from build123d import *

# Parameters (mm, degrees)
EXTRUDE_1_DEPTH     = 42.5
SKETCH_2_OUTSIDE_W  = 122.554
SKETCH_2_OUTSIDE_H  = 44.054
CUT_EXTRUDE_1_DEPTH = 78
SKETCH_3_W          = 40
SKETCH_3_H          = 40
CUT_EXTRUDE_2_DEPTH = 7.5
SKETCH_4_W          = 152
SKETCH_4_H          = 82
CUT_EXTRUDE_3_DEPTH = 2


with BuildPart() as part:
    # Эскиз1 → Бобышка-Вытянуть1 (new body, symmetric)
    with BuildSketch(Plane.XY):
        Polygon((0, 0), (-78, 0), (-78, 2.705180544), (-60.423159652, 6.5), (-10.423159652, 6.5), (0, 2.705180544), (10.423159652, 6.5), (60.423159652, 6.5), (78, 2.705180544), (78, 0), align=None)
    extrude(amount=EXTRUDE_1_DEPTH, both=True)

    # Эскиз2 outside → Вырез-Вытянуть1 (cut, symmetric)
    with BuildSketch(Plane(origin=(0, 0, 0), x_dir=(0, 0, -1), z_dir=(1, 0, 0))):
        with Locations((0, 3.25)):
            Rectangle(SKETCH_2_OUTSIDE_W, SKETCH_2_OUTSIDE_H)
        Polygon((42.5, 0), (-42.5, 0), (-42.5, 2.705180544), (-22.5, 6.5), (22.5, 6.5), (42.5, 2.705180544), align=None, mode=Mode.SUBTRACT)
    extrude(amount=CUT_EXTRUDE_1_DEPTH, both=True, mode=Mode.SUBTRACT)

    # Эскиз3 → Вырез-Вытянуть2 (cut, through all)
    with BuildSketch(Plane.XZ):
        with Locations((-35.5, 0)):
            Rectangle(SKETCH_3_W, SKETCH_3_H)
        with Locations((35.5, 0)):
            Rectangle(SKETCH_3_W, SKETCH_3_H)
    extrude(amount=-CUT_EXTRUDE_2_DEPTH, mode=Mode.SUBTRACT)

    # Эскиз4 → Вырез-Вытянуть3 (cut)
    with BuildSketch(Plane.XZ):
        Rectangle(SKETCH_4_W, SKETCH_4_H)
    extrude(amount=-CUT_EXTRUDE_3_DEPTH, mode=Mode.SUBTRACT)


solid = part.part
Geometry: final body of the model. Coordinates: model frame, mm. A direction names the side the tool comes from. Round coordinates to 2 decimals unless told otherwise and drop trailing zeros. Loops run counter-clockwise (first coordinate to the right, second up) from the corner with the lowest first, then second, coordinate; pieces in that order, holes last. Notation, with made-up numbers: M 23,-2 L 30,-2 A12 cw 30,12 Z; hole C 43.5,87.5 d5. An arc over 180 degrees is marked long. Put each result on its own line as item: value. Start each with the question number.
(1) Section query B-B (x = -24). Return loops of the section in (y, z), then the cut area to 3 significant figures.
(2) Set-up query: faces 5 (the face through (-36, 4, 20)), 6 (the face through (-69.335, 4.576, 0.595)), 7 (the face through (5.139, 4.576, 0.595)). Return all of +Z, -Z, +X, -X, +Y, -Y with unobstructed straight access to the full face (end or side cutting, diameter ignored); none if empty.
(3) Draft query along X for faces 1 (the face through (69.09, 4.63, 0.59)), 2 (the face through (-1, 2, 1)), 3 (the face through (-5.285, 4.629, 0.595)), 4 (the face through (39.55, 4.63, -32.36)). Return one class per face: +X half, -X half, draft (parallel to the pull), parting line (faces both ways), or undercut.
(4) Material intervals for line 1 along X through (y, z) = (0.5, 26); line 2 along Z through (x, y) = (44, 0.75); line 3 along Z through (x, y) = (-48.5, 2.5), sorted ascending. Write a range as [from, to].
(5) Section query D-D (x = 57). Return loops of the section in (y, z).
(6) Section query C-C (z = -4). Return loops of the section in (x, y).
(7) Section query A-A (y = 5). Return loops of the section in (x, z).
(8) Contact query for a flat-ended pin moving along its axis: pin 1 Ø24.5 at (x, z) = (6.5, 20.5) entering from -Y. Output: stop coordinate, or through.
Findings below:
1. outline: M 0,-42.5 L 2.71,-42.5 L 6.5,-22.5 L 6.5,-20 L 2,-20 L 2,-41 L 0,-41 Z; M 0,41 L 2,41 L 2,20 L 6.5,20 L 6.5,22.5 L 2.71,42.5 L 0,42.5 Z
1. area: 133 mm2
2. face 5: +Y, -Y
2. face 6: +Z, -Z, -X, +Y
2. face 7: +Z, -Z, +Y
3. face 1: +X half
3. face 2: undercut
3. face 3: undercut
3. face 4: draft
4. line 1: x = [-78, -76], [76, 78]
4. line 2: z = [-42.5, -41], [41, 42.5]
4. line 3: z = [-42.5, -20], [20, 42.5]
5. outline: M 0,-42.5 L 2.71,-42.5 L 6.5,-22.5 L 6.5,22.5 L 2.71,42.5 L 0,42.5 L 0,41 L 2,41 L 2,-41 L 0,-41 Z
6. outline: M -78,0 L -76,0 L -76,2 L -55.5,2 L -55.5,6.5 L -60.42,6.5 L -78,2.71 Z; M -15.5,2 L 15.5,2 L 15.5,6.5 L 10.42,6.5 L 0,2.71 L -10.42,6.5 L -15.5,6.5 Z; M 55.5,2 L 76,2 L 76,0 L 78,0 L 78,2.71 L 60.42,6.5 L 55.5,6.5 Z
7. outline: M -67.37,-30.41 L -6.3,-30.41 L -6.3,30.41 L -67.37,30.41 Z; M 6.3,-30.41 L 67.37,-30.41 L 67.37,30.41 L 6.3,30.41 Z; hole M -55.5,-20 L -15.5,-20 L -15.5,20 L -55.5,20 Z; hole M 15.5,-20 L 55.5,-20 L 55.5,20 L 15.5,20 Z
8. pin 1: stops at y = 2
